Read the model definition and answer for the solid it produces. Units are mm, in the model's axes. A direction names the side the tool comes from. Coordinates: 2 decimals unless noted, no trailing zeros. Order: outer loops, then holes, each group sorted by start corner. A loop starts at its lowest first (then second) coordinate and runs counter-clockwise, first axis right, second up. Notation, with made-up numbers: M 56,15.5 L 69,15.5 A15 ccw 69,19.5 Z; hole C 84,37.5 d3. An arc over 180 degrees is marked long. Use a Markdown table: item, result. Add a question column.
1) Find section A-A on y = -31.5. Write down the section's boundary in (x, z).
2) For faces 5 (the face through (-17, 20, 7)), 6 (the face through (-39.778, -0.28, -21.057)), 7 (the face through (25, 0, 20)), determine the directions among +Z, -Z, +X, -X, +Y, -Y from which every point of the face is accessible in a straight line to the end or side of a thin tool.
3) The mould has two halves that part along Z. Classify faces 1 (the face through (-5, -45, 0)), 2 (the face through (-17, -12, -30)), 3 (the face through (-18.49, -2.38, 15.91)), 4 (the face through (-3, -32, 0)): released by +Z, released by -Z, zero draft, split by the parting line, or undercut.
4) Find section D-D on z = -11. Write down the section's boundary in (x, y).
5) Find section C-C on z = 0. Write down the section's boundary in (x, y).
6) Each of these flat-tipped pins is pushed along its axis until it touches: pin 1 Ø7 at (x, z) = (0, 0) entering from -Y; pin 2 Ø2 at (y, z) = (-15, -13) entering from -X; pin 3 Ø3 at (y, z) = (-32.5, -9) entering from -X; pin 4 Ø12 at (y, z) = (-5.5, -11.5) entering from +X. Where does it stop, or does it pass through?
7) Find the intervals of material crossed by probe 1 along Z at (x, y) = (-14, -11); probe 2 along Z at (x, y) = (0, -29); probe 3 along Y at (x, z) = (10.5, 3.5), in increasing order. Write a range as [from, to].
8) Find section B-B on x = 11. Write down the section's boundary in (y, z), plus the area to 3 significant figures.
from build123d import *

# Parameters (mm, degrees)
PAD_DEPTH    = 20
SKETCH001_R  = 3
PAD001_DEPTH = 25
SKETCH002_R  = 3
POCKET_DEPTH = 79.427407
FILLET_R     = 2
FILLET001_R  = 3


with BuildPart() as part:
    # Sketch → Pad (new body, symmetric)
    with BuildSketch(Plane.XZ):
        with BuildLine():
            Line((0.908117, 17.87868), (-34.849242, -17.87868))
            ThreePointArc((-34.849242, -17.87868), (-39.742201, -21.14805), (-33.970563, -20))
            Line((-33.970563, -20), (43.029437, -20))
            Line((43.029437, -20), (43.029437, -30))
            Line((43.029437, -30), (-82.325902, -30))
            Line((-22.325902, 30), (-82.325902, -30))
            Line((43.029437, 30), (-22.325902, 30))
            Line((43.029437, 20), (43.029437, 30))
            Line((6.029437, 20), (43.029437, 20))
            ThreePointArc((6.029437, 20), (1.881387, 22.771639), (0.908117, 17.87868))
        make_face()
    extrude(amount=PAD_DEPTH, both=True)

    # Sketch001 → Pad001 (join)
    with BuildSketch(Plane.XZ.offset(20)):
        Polygon((43.029437, -20), (43.029437, 20), (43.029437, 30), (-22.325902, 30), (-82.325902, -30), (43.029437, -30), align=None)
        Circle(SKETCH001_R, mode=Mode.SUBTRACT)
    extrude(amount=PAD001_DEPTH)

    # Sketch002 → Pocket (cut, through all)
    with BuildSketch(Plane(origin=(0, 0, 0), x_dir=(0, 1, 0), z_dir=(0.707107, 0, -0.707107))):
        Circle(SKETCH002_R)
    extrude(amount=-POCKET_DEPTH, mode=Mode.SUBTRACT)

    # Fillet
    fillet_edges = [part.edges().sort_by_distance(p)[0] for p in [
        (-33.970563, 0, -20),
        (-34.849242, 0, -17.87868),
        (0.908117, 0, 17.87868),
        (6.029437, 0, 20),
    ]]
    fillet(fillet_edges, radius=FILLET_R)

    # Fillet001
    fillet001_edges = [part.edges().sort_by_distance(p)[0] for p in [
        (-82.325902, -32.5, -30),
        (-82.325902, 0, -30),
    ]]
    fillet(fillet001_edges, radius=FILLET001_R)


solid = part.part
Check result:
| question | item | result |
|---|---|---|
| 1 | outline | M -77.2,-24.88 A3 ccw -75.08,-30 L 43.03,-30 L 43.03,30 L -22.33,30 Z; hole C 0,0 d6 |
| 2 | face 5 | +Z, -Z, +X, -X, +Y |
| 2 | face 6 | +Y |
| 2 | face 7 | +X, +Y |
| 3 | face 1 | zero draft |
| 3 | face 2 | released by -Z |
| 3 | face 3 | undercut |
| 3 | face 4 | undercut |
| 4 | outline | M -63.33,-45 L 43.03,-45 L 43.03,-20 L -27.97,-20 L -27.97,20 L -63.33,20 Z |
| 5 | outline | M -52.33,-45 L -3,-45 L -3,-20 L -16.97,-20 L -16.97,20 L -52.33,20 Z; M 3,-45 L 43.03,-45 L 43.03,-20 L 3,-20 Z |
| 6 | pin 1 | stops at y = -45 |
| 6 | pin 2 | stops at x = -66.33 |
| 6 | pin 3 | stops at x = -62.83 |
| 6 | pin 4 | stops at x = -22.47 |
| 7 | probe 1 | z = [-30, -20], [2.97, 30] |
| 7 | probe 2 | z = [-30, -3], [3, 30] |
| 7 | probe 3 | y = [-45, -20] |
| 8 | outline | M -45,-30 L 20,-30 L 20,-20 L -20,-20 L -20,20 L 20,20 L 20,30 L -45,30 Z |
| 8 | area | 2,300 mm2 |
